```python
from build123d import *

# Parameters (mm, degrees)
SKETCH1_W           = 80
SKETCH1_H           = 40
SKETCH1_R           = 2.55
SKETCH1_R_2         = 10
SKETCH1_R_3         = 1.325
BOSS_EXTRUDE1_DEPTH = 3.175


with BuildPart() as part:
    # Sketch1 → Boss-Extrude1 (new body)
    with BuildSketch(Plane(origin=(0, 0, 0), x_dir=(1, 0, 0), z_dir=(0, 1, 0))):
        with Locations((40, 20)):
            Rectangle(SKETCH1_W, SKETCH1_H)
        with Locations((54, 20)):
            Circle(SKETCH1_R, mode=Mode.SUBTRACT)
        with Locations((74, 20)):
            Circle(SKETCH1_R, mode=Mode.SUBTRACT)
        with Locations((19, 20)):
            Circle(SKETCH1_R_2, mode=Mode.SUBTRACT)
        with Locations((28.192388155, 10.807611845)):
            Circle(SKETCH1_R_3, mode=Mode.SUBTRACT)
        with Locations((9.807611845, 10.807611845)):
            Circle(SKETCH1_R_3, mode=Mode.SUBTRACT)
        with Locations((9.807611845, 29.192388155)):
            Circle(SKETCH1_R_3, mode=Mode.SUBTRACT)
        with Locations((28.192388155, 29.192388155)):
            Circle(SKETCH1_R_3, mode=Mode.SUBTRACT)
    extrude(amount=BOSS_EXTRUDE1_DEPTH)


solid = part.part
```
Verification items for the finished model (mm, model axes). Give positions to 0.01 mm unless a question says otherwise; leave off trailing zeros. Order: outer loops, then holes, each group sorted by start corner. A loop starts at its lowest first (then second) coordinate and runs counter-clockwise, first axis right, second up. Notation, with made-up numbers: M 49,37 L 85,37 A23 ccw 85,70 Z; hole C -1.75,-21 d1. An arc over 180 degrees is marked long. Answer in a Markdown table with one row per item. Add a question column.
Item 1: Section check A-A, the plane x = 54. Enter the section's corners in (y, z) (3 decimals).
Item 2: Section check C-C, the plane y = 0.6. Enter the section's corners in (x, z) (3 decimals), and give its area (3 significant figures).
Item 3: Mould release check, pull along Z, two halves, no side actions. Record for faces 1 (the cylindrical face through (26.87, 1.57, -10.87)), 2 (the flat face through (39, 2, -40)), 3 (the flat face through (39, 2, 0)), 4 (the flat face through (39, 0, -20)): released by +Z, released by -Z, zero draft, split by the parting line, or undercut.
Item 4: Scan lines: probe 1 along Z at (x, y) = (19, 1.9); probe 2 along X at (y, z) = (2, -20); probe 3 along X at (y, z) = (1.7, -11.5). Record each from-to range of solid material in increasing order. Write a range as from..to.
Item 5: Section check B-B, the plane z = -20. Enter the section's corners in (x, y) (3 decimals), and give its area (3 significant figures).
Item 6: Section check D-D, the plane z = -13. Enter the section's corners in (x, y) (3 decimals), and give its area (3 significant figures).
Filled sheet:
| question | item | result |
|---|---|---|
| 1 | outline | M 0,-40 L 3.175,-40 L 3.175,-22.55 L 0,-22.55 Z; M 0,-17.45 L 3.175,-17.45 L 3.175,0 L 0,0 Z |
| 2 | outline | M 0,-40 L 80,-40 L 80,0 L 0,0 Z; hole C 9.808,-29.192 d2.65; hole C 9.808,-10.808 d2.65; hole C 19,-20 d20; hole C 28.192,-29.192 d2.65; hole C 28.192,-10.808 d2.65; hole C 54,-20 d5.1; hole C 74,-20 d5.1 |
| 2 | area | 2,820 mm^2 |
| 3 | face 1 | undercut |
| 3 | face 2 | released by -Z |
| 3 | face 3 | released by +Z |
| 3 | face 4 | zero draft |
| 4 | probe 1 | z = -40..-30, -10..0 |
| 4 | probe 2 | x = 0..9, 29..51.45, 56.55..71.45, 76.55..80 |
| 4 | probe 3 | x = 0..8.68, 10.94..13.73, 24.27..27.06, 29.32..80 |
| 5 | outline | M 0,0 L 9,0 L 9,3.175 L 0,3.175 Z; M 29,0 L 51.45,0 L 51.45,3.175 L 29,3.175 Z; M 56.55,0 L 71.45,0 L 71.45,3.175 L 56.55,3.175 Z; M 76.55,0 L 80,0 L 80,3.175 L 76.55,3.175 Z |
| 5 | area | 158 mm^2 |
| 6 | outline | M 0,0 L 11.859,0 L 11.859,3.175 L 0,3.175 Z; M 26.141,0 L 80,0 L 80,3.175 L 26.141,3.175 Z |
| 6 | area | 209 mm^2 |
